Check sheet for the modelled part. Datum: model origin and axes. Units: mm. A direction names the side the tool comes from. Coordinates: 2 decimals unless noted, no trailing zeros. Loops run counter-clockwise (first coordinate to the right, second up) from the corner with the lowest first, then second, coordinate; pieces in that order, holes last. Notation, with made-up numbers: (-29, 45.5) -> (24, 45.5) arc R15 ccw to (24, 61.5) -> close; hole circle Ø8 at (66.25, 49.5). An arc over 180 degrees is marked (long way). Use CSV: the item, a comma, the result in double quotes.
Autodesk Inventor part; units mm, degrees
ref_plane "YZ Plane" through (0, 0, 0) normal (1, 0, 0) x (0, 1, 0)
ref_plane "XZ Plane" through (0, 0, 0) normal (0, 1, 0) x (-1, 0, 0)
ref_plane "XY Plane" through (0, 0, 0) normal (0, 0, 1) x (1, 0, 0)
sketch "Skizze1" plane through (0, 0, 0) normal (0, 1, 0) x (-1, 0, 0)
  line L0 (-100, 15) -> (100, 15)
  line L1 (100, 15) -> (100, -15)
  line L2 (100, -15) -> (-100, -15)
  line L3 (-100, -15) -> (-100, 15)
  line L4 (-100, 15) -> (100, -15) construction
  line L5 (100, 15) -> (-100, -15) construction
  point P0 (0, 0)
  dimension "d0" = 30
  dimension "d1" = 200
extrude "Extrusion1" add sketch "Skizze1" along normal blind 10
sketch "Skizze4" plane through (0, 10, 0) normal (0, 1, 0) x (1, 0, 0)
  line L0 (100, 15) -> (-100, 15)
  line L1 (100, -15) -> (100, 15)
  line L2 (-100, -15) -> (100, -15)
  line L3 (-100, 15) -> (-100, -15)
  line L4 (0, 21) -> (0, -21)
  point P0 (0, 0)
  point P1 (6.25, 7.5)
  point P2 (6.25, -7.5)
  point P3 (-6.25, -7.5)
  point P4 (-6.25, 7.5)
  dimension "d37" = 7.5
  dimension "d40" = 7.5
  dimension "d41" = 7.5
  dimension "d44" = 7.5
  dimension "d52" = 6.25
  dimension "d53" = 6.25
  dimension "d54" = 6.25
  dimension "d55" = 6.25
hole "Bohrung3" at (6.25, 10, -7.5) at (6.25, 10, 7.5) at (-6.25, 10, 7.5) at (-6.25, 10, -7.5) direction (0, -1, 0) diameter 4.134 depth 14.2
sketch "Skizze5" plane through (0, 0, 0) normal (0, -1, 0) x (1, 0, 0)
  line L0 (-100, 15) -> (100, 15)
  line L1 (-70, -15) -> (-100, -15)
  line L2 (-100, -15) -> (-100, 15)
  line L3 (-100, 15) -> (-70, 15)
  line L4 (-70, 15) -> (-70, -15)
  line L5 (-70, -15) -> (-100, 15) construction
  line L6 (-100, -15) -> (-70, 15) construction
  line L7 (-100, -15) -> (-100, 15)
  line L8 (100, -15) -> (-100, -15)
  line L9 (70, -15) -> (100, -15)
  line L10 (100, -15) -> (100, 15)
  line L11 (100, 15) -> (70, 15)
  line L12 (70, 15) -> (70, -15)
  line L13 (70, -15) -> (100, 15) construction
  line L14 (100, -15) -> (70, 15) construction
  line L15 (100, 15) -> (100, -15)
  point P0 (0, 0)
  point P1 (-12.5, 15)
  point P2 (-85, 0)
  point P3 (-12.5, -15)
  point P4 (85, 0)
  dimension "d56" = 0
  dimension "d57" = 0
  dimension "d58" = 30
  dimension "d59" = 30
  dimension "d60" = 30
  dimension "d61" = 0
extrude "Extrusion3" add sketch "Skizze5" along normal blind 30 contours L0 L4 L1 L2 | L0 L10 L8 L12
sketch "Skizze6" plane through (0, -30, 0) normal (0, -1, 0) x (1, 0, 0)
  line L0 (-110, -25) -> (-60, -25)
  line L1 (-60, -25) -> (-60, 25)
  line L2 (-60, 25) -> (-110, 25)
  line L3 (-110, 25) -> (-110, -25)
  line L4 (-110, -25) -> (-60, 25) construction
  line L5 (-60, -25) -> (-110, 25) construction
  line L6 (-70, -15) -> (-70, 15)
  line L7 (60, 25) -> (110, 25)
  line L8 (110, 25) -> (110, -25)
  line L9 (110, -25) -> (60, -25)
  line L10 (60, -25) -> (60, 25)
  line L11 (60, 25) -> (110, -25) construction
  line L12 (110, 25) -> (60, -25) construction
  line L13 (100, -15) -> (100, 15)
  point P0 (0, 0)
  point P1 (-85, 0)
  point P2 (85, 0)
  dimension "d64" = 15
  dimension "d65" = 50
  dimension "d66" = 50
  dimension "d67" = 15
  dimension "d86" = 50
  dimension "d87" = 50
extrude "Extrusion4" add sketch "Skizze6" along normal blind 10
fillet "Rundung1" radius 5 8 edges at (-110, -35, 25) (-60, -35, 25) (-110, -35, -25) (-60, -35, -25) (60, -35, -25) (110, -35, -25) (110, -35, 25) (60, -35, 25)
sketch "Skizze7" plane through (0, -30, 0) normal (0, 1, 0) x (1, 0, 0)
  line L0 (110, 20) -> (110, -20)
  line L1 (105, -25) -> (65, -25)
  line L2 (60, -20) -> (60, 20)
  line L3 (65, 25) -> (105, 25)
  line L4 (-60, 20) -> (-60, -20)
  line L5 (-65, -25) -> (-105, -25)
  line L6 (-110, -20) -> (-110, 20)
  line L7 (-105, 25) -> (-65, 25)
  point P0 (0, 0)
  point P1 (104, -19)
  point P2 (66, -19)
  point P3 (66, 19)
  point P4 (104, 19)
  point P5 (-66, -19)
  point P6 (-104, -19)
  point P7 (-104, 19)
  point P8 (-66, 19)
  dimension "d71" = 6
  dimension "d72" = 6
  dimension "d73" = 6
  dimension "d74" = 6
  dimension "d75" = 6
  dimension "d76" = 6
  dimension "d77" = 6
  dimension "d78" = 6
  dimension "d79" = 6
  dimension "d80" = 6
  dimension "d81" = 6
  dimension "d82" = 6
  dimension "d83" = 6
  dimension "d84" = 6
  dimension "d85" = 6
  dimension "d95" = 6
hole "Bohrung4" at (-66, -30, 19) at (104, -30, 19) at (104, -30, -19) at (66, -30, -19) at (66, -30, 19) at (-104, -30, 19) at (-66, -30, -19) at (-104, -30, -19) direction (0, -1, 0) diameter 4.134 depth 14.2
fillet "Rundung2" radius 5 4 edges at (100, 10, 0) (-100, 10, 0) (70, 0, 0) (-70, 0, 0)
equation "\"d46\" = d42"
equation "\"d89\" = d83"
properties part number "Platte für Gehäuse" material "Stahl"
1) Cross-section at C-C on y = -33. Give the number of separate pieces and of enclosed holes in the cut face, and give its area (3 significant figures).
Answer below:
separate pieces,"2"
enclosed holes,"8"
area,"4,850 mm²"
2) Cross-section at A-A on y = -21. Record the boundary of the cut face in (x, z).
Answer below:
outline,"(-100, -15) -> (-70, -15) -> (-70, 15) -> (-100, 15) -> close; (70, -15) -> (100, -15) -> (100, 15) -> (70, 15) -> close"
3) Access from +Z, -Z, +X, -X, +Y, -Y to the whole of each face (thin tool, end or side, straight path). Record for faces 5 (the cylindrical face through (68, -1, 0)), 6 (the flat face through (-85, -35, 25)), 7 (the cylindrical face through (62, -35, 24)), 8 (the flat face through (-1, 3, -15)).
Answer below:
face 5,"+Z, -Z"
face 6,"+Z, +X, -X, +Y, -Y"
face 7,"+Z, +Y, -Y"
face 8,"-Z, +X, -X, +Y"
4) Thickness scan on line 1 along Z through (x, y) = (-66, -33.5); line 2 along X through (y, z) = (-36.5, 19); line 3 along X through (y, z) = (2.25, -7.5). Record the ranges inside material, lowest first. Write a range as from..to.
Answer below:
line 1,"z = -25..-21.07, -16.93..16.93, 21.07..25"
line 2,"x = -110..-106.07, -101.93..-68.07, -63.93..-60, 60..63.93, 68.07..101.93, 106.07..110"
line 3,"x = -100..-8.32, -4.18..4.18, 8.32..100"
5) Cross-section at D-D on x = -6.25. Record the boundary of the cut face in (y, z).
Answer below:
outline,"(0, -15) -> (10, -15) -> (10, -9.57) -> (0, -9.57) -> close; (0, -5.43) -> (10, -5.43) -> (10, 5.43) -> (0, 5.43) -> close; (0, 9.57) -> (10, 9.57) -> (10, 15) -> (0, 15) -> close"
6) Cross-section at B-B on z = 7.5. Record the boundary of the cut face in (x, y), and give its area (3 significant figures).
Answer below:
outline,"(-110, -40) -> (-60, -40) -> (-60, -30) -> (-70, -30) -> (-70, -5) arc R5 cw to (-65, 0) -> (-8.32, 0) -> (-8.32, 10) -> (-95, 10) arc R5 ccw to (-100, 5) -> (-100, -30) -> (-110, -30) -> close; (-4.18, 0) -> (4.18, 0) -> (4.18, 10) -> (-4.18, 10) -> close; (8.32, 0) -> (65, 0) arc R5 cw to (70, -5) -> (70, -30) -> (60, -30) -> (60, -40) -> (110, -40) -> (110, -30) -> (100, -30) -> (100, 5) arc R5 ccw to (95, 10) -> (8.32, 10) -> close"
area,"4,720 mm²"
7) Draft check along Z on faces 1 (the cylindrical face through (4.85, 4.93, -9.02)), 2 (the cylindrical face through (61, -35, -23)), 3 (the flat face through (1, 3, 15)), 4 (the flat face through (-60, -35, 0)). Enter one of: released by +Z, released by -Z, zero draft, split by the parting line, or undercut.
Answer below:
face 1,"undercut"
face 2,"released by -Z"
face 3,"released by +Z"
face 4,"zero draft"
8) Go/stop test with flat-tipped pins: pin 1 Ø5 at (y, z) = (-16, -9.5) entering from +X; pin 2 Ø3.5 at (x, z) = (-104, 19) entering from -Y; pin 3 Ø7.5 at (y, z) = (-21, 2.5) entering from -X; pin 4 Ø15 at (x, z) = (96, -7) entering from +Y. Record where each tip stops, or that it passes through.
Answer below:
pin 1,"stops at x = 100"
pin 2,"passes through"
pin 3,"stops at x = -100"
pin 4,"stops at y = 10"
